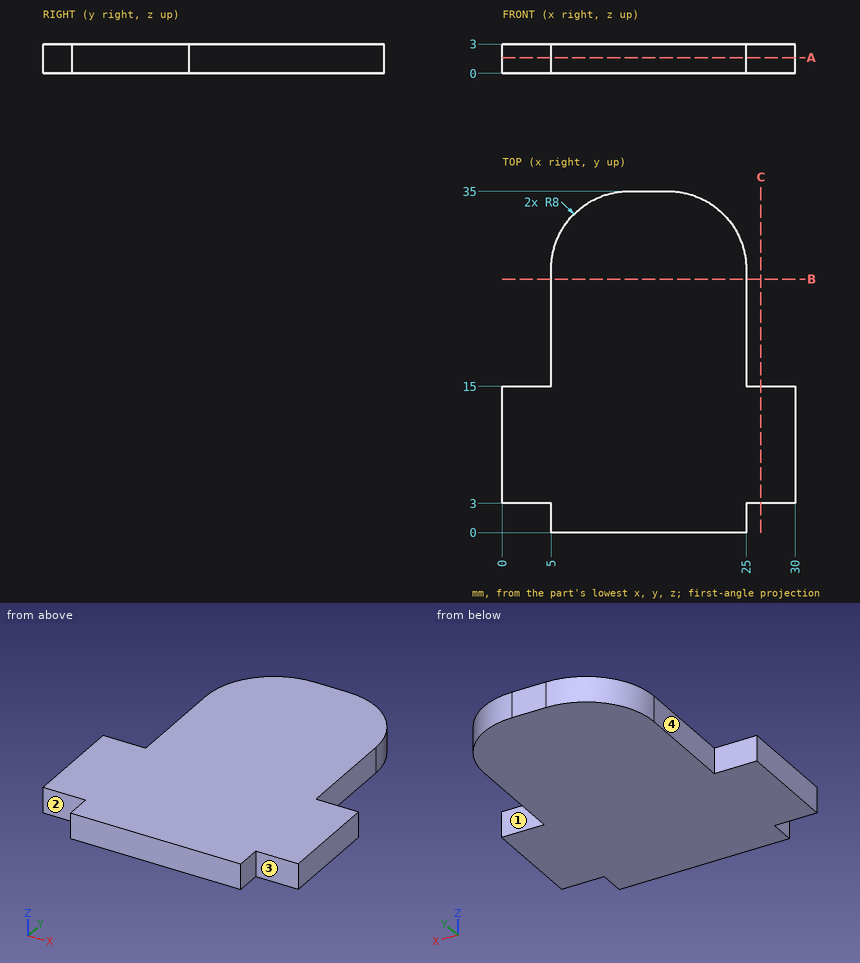
Could you check a few things on this drawing? It's one solid part, dimensions in mm from its lowest x, y, z. A direction names the side the tool comes from. Give positions to 0.01 mm unless a question says otherwise; leave off trailing zeros. Order: outer loops, then holes, each group sorted by start corner. A loop starts at its lowest first (then second) coordinate and runs counter-clockwise, first axis right, second up. Notation, with made-up numbers: (-38, 15.25) - (-26, 15.25) arc R22 cw to (-26, 42.25) - close; hole circle Ø5 at (58, -6). An arc over 180 degrees is marked (long way). Answer as a JSON object with one key per item and string values. Group by question number.
Item 1: Which directions (+Z, -Z, +X, -X, +Y, -Y) give clear straight access to the entire face, cutting with the end or side of a thin tool? Please do the marked faces 1, 2, 3 and 4.
Item 2: If we section it at A-A on z = 1.6: Please give me the cut outline in (x, y), and give its area (3 significant figures).
Item 3: For P1, Ø0.9, axis at y = 2, z = 1.5, coming from the +X side; P2, Ø0.9, axis at y = 22.5, z = 2, coming from the -X side; P3, Ø1.5, axis at x = 28.5, z = 1, coming from the -Y side, each with a flat end and sliding along its axis, tell me the tip position at first contact or that it passes through.
Item 4: Please list where these lines run through material, in increasing order: probe 1 along X at (y, z) = (20.5, 1.65); probe 2 along Y at (x, z) = (26.25, 2.4); probe 3 along Y at (x, z) = (19, 1.6).
Item 5: If we section it at B-B on y = 26: Please give me the cut outline in (x, z).
Item 6: If we section it at C-C on x = 26.5: Please give me the cut outline in (y, z), and give its area (3 significant figures).
Result set:
{
 "1": {"face 1": "+Z, -Z, +X, +Y", "face 2": "+Z, -Z, -X, -Y", "face 3": "+Z, -Z, +X, -Y", "face 4": "+Z, -Z, -X, +Y"},
 "2": {"outline": "(0, 3) - (5, 3) - (5, 0) - (25, 0) - (25, 3) - (30, 3) - (30, 15) - (25, 15) - (25, 27) arc R8 ccw to (17, 35) - (13, 35) arc R8 ccw to (5, 27) - (5, 15) - (0, 15) - close", "area": "793 mm²"},
 "3": {"P1": "x = 25", "P2": "x = 5", "P3": "y = 3"},
 "4": {"probe 1": "5 to 25", "probe 2": "3 to 15", "probe 3": "0 to 34.75"},
 "5": {"outline": "(5, 0) - (25, 0) - (25, 3) - (5, 3) - close"},
 "6": {"outline": "(3, 0) - (15, 0) - (15, 3) - (3, 3) - close", "area": "36.0 mm²"}
}
